For this review, take the finished solid that the model builds, in its own axes (mm). A direction names the side the tool comes from. Give positions to 0.01 mm unless a question says otherwise; leave off trailing zeros. Order: outer loops, then holes, each group sorted by start corner. A loop starts at its lowest first (then second) coordinate and runs counter-clockwise, first axis right, second up. Notation, with made-up numbers: M 82.25,-15.75 L 129.25,-15.75 A24 ccw 129.25,-4.75 Z; hole C 83,-15.75 d10. An arc over 180 degrees is marked long. Use CSV: the item, a comma, the result in double quotes. Start each with the question number.
(1) Draft analysis for pull direction Y (two halves, no side actions). For faces 1 (the face through (114.619, 88.085, 140.14)), 2 (the face through (-3, -100, 74)), 3 (the face through (200, -1, 74)), state which applies: pulls with the +Y half, pulls with the -Y half, needs draft (parallel to the pull), parting line crosses it, or undercut.
(2) Consider section A-A (z = 41). Write out the cut boundary in (x, y), and give its area (3 significant figures).
(3) Consider section C-C (y = -26). Write out the cut boundary in (x, z).
(4) Tool access review of faces 4 (the face through (-200, -1, 74)), 5 (the face through (-3, 19, 20)): name each direction out of +Z, -Z, +X, -X, +Y, -Y from which nothing blocks a thin tool from reaching the whole face with its end or side.
(5) Consider section B-B (x = -110). Write out the cut boundary in (y, z).
(6) Clearance check with a flat-ended pin moving along its axis: P1, Ø1.5, axis at x = -46.5, y = 46.5, coming from the +Z side. State where the tip first meets the part, or that it passes through.
(7) Wall thickness on L1, parallel to Y at x = 110, z = 143; L2, parallel to X at y = -18, z = 25; L3, parallel to Y at x = -158, z = 112: over which ranges is each line inside the solid? List them lowest first. Write a range as from..to.
(8) Consider section D-D (x = 94). Write out the cut boundary in (y, z), and give its area (3 significant figures).
```python
from build123d import *

# Parameters (mm, degrees)
F0_W     = 400
F0_H     = 200
F1_DEPTH = 150
F2_W     = 360
F2_H     = 160
F3_DEPTH = 130
F4_R     = 5
F5_DEPTH = 20
F7_D     = 10
F7_DEPTH = 7
F7_TIP   = 3.0043030951


with BuildPart() as f1:
    # F0 (on Top) → F1 (new body)
    with BuildSketch(Plane.XY):
        Rectangle(F0_W, F0_H)
    extrude(amount=F1_DEPTH)

    # F2 (on face) → F3 (cut)
    with BuildSketch(Plane.XY.offset(150)):
        Rectangle(F2_W, F2_H)
    extrude(amount=-F3_DEPTH, mode=Mode.SUBTRACT)

    # F4 (on face) → F5 (cut)
    with BuildSketch(Plane.XY.offset(150)):
        with Locations((-150, 90)):
            Circle(F4_R)
        with Locations((-110, 90)):
            Circle(F4_R)
        with Locations((110, 90)):
            Circle(F4_R)
        with Locations((150, 90)):
            Circle(F4_R)
    extrude(amount=-F5_DEPTH, mode=Mode.SUBTRACT)

    # F7
    with Locations(Plane.XY.offset(20)):
        with Locations((0, 0)):
            Hole(F7_D / 2, depth=F7_DEPTH)
            with Locations((0, 0, -(F7_DEPTH + F7_TIP / 2))):  # 118° drill point
                Cone(0, F7_D / 2, F7_TIP, mode=Mode.SUBTRACT)


solid = f1.part
```
Check result:
1,face 1,"undercut"
1,face 2,"pulls with the -Y half"
1,face 3,"needs draft"
2,outline,"M -200,-100 L 200,-100 L 200,100 L -200,100 Z; hole M -180,-80 L 180,-80 L 180,80 L -180,80 Z"
2,area,"22,400 mm^2"
3,outline,"M -200,0 L 200,0 L 200,150 L 180,150 L 180,20 L -180,20 L -180,150 L -200,150 Z"
4,face 4,"+Z, -Z, -X, +Y, -Y"
4,face 5,"+Z"
5,outline,"M -100,0 L 100,0 L 100,150 L 95,150 L 95,130 L 85,130 L 85,150 L 80,150 L 80,20 L -80,20 L -80,150 L -100,150 Z"
6,P1,"stops at z = 20"
7,L1,"y = -100..-80, 80..85, 95..100"
7,L2,"x = -200..-180, 180..200"
7,L3,"y = -100..-80, 80..100"
8,outline,"M -100,0 L 100,0 L 100,150 L 80,150 L 80,20 L -80,20 L -80,150 L -100,150 Z"
8,area,"9,200 mm^2"
